```python
from build123d import *

# Parameters (mm, degrees)
REVOLVE1_ANGLE                                       = 180
BOSS_EXTRUDE1_DEPTH                                  = 10
BOSS_EXTRUDE1_DEPTH_BACK                             = 10
SKETCH2_W                                            = 5
SKETCH2_H                                            = 20
CUT_EXTRUDE1_DEPTH                                   = 10
CSK_FOR_M1_6_COUNTERSUNK_FLAT_HEAD_SCREW_D           = 1.8
CSK_FOR_M1_6_COUNTERSUNK_FLAT_HEAD_SCREW_DEPTH       = 5
CSK_FOR_M1_6_COUNTERSUNK_FLAT_HEAD_SCREW_CSINK_D     = 3.6
CSK_FOR_M1_6_COUNTERSUNK_FLAT_HEAD_SCREW_CSINK_ANGLE = 90
CSK_FOR_M1_6_COUNTERSUNK_FLAT_HEAD_SCREW_TIP         = 0.540774557
CSK_FOR_M1_6_COUNTERSUNK_FLAT_HEAD_S_2_D             = 1.8
CSK_FOR_M1_6_COUNTERSUNK_FLAT_HEAD_S_2_DEPTH         = 5
CSK_FOR_M1_6_COUNTERSUNK_FLAT_HEAD_S_2_CSINK_D       = 3.6
CSK_FOR_M1_6_COUNTERSUNK_FLAT_HEAD_S_2_CSINK_ANGLE   = 90
CSK_FOR_M1_6_COUNTERSUNK_FLAT_HEAD_S_2_TIP           = 0.540774557
CSK_FOR_M1_6_COUNTERSUNK_FLAT_HEAD_S_3_D             = 1.8
CSK_FOR_M1_6_COUNTERSUNK_FLAT_HEAD_S_3_DEPTH         = 5
CSK_FOR_M1_6_COUNTERSUNK_FLAT_HEAD_S_3_CSINK_D       = 3.6
CSK_FOR_M1_6_COUNTERSUNK_FLAT_HEAD_S_3_CSINK_ANGLE   = 90
CSK_FOR_M1_6_COUNTERSUNK_FLAT_HEAD_S_3_TIP           = 0.540774557
SKETCH9_R                                            = 3
CUT_EXTRUDE2_DEPTH                                   = 3
CUT_EXTRUDE3_START                                   = -3
SKETCH10_R                                           = 3
CUT_EXTRUDE3_DEPTH                                   = 3


with BuildPart() as part:
    # Sketch1 → Revolve1 (revolve)
    with BuildSketch(Plane.XY):
        with BuildLine():
            Line((61, 170), (61, 0))
            Line((61, 0), (58, 0))
            Line((58, 0), (58, 170))
            ThreePointArc((58, 170), (41.873834296, 218.154039035), (0, 246.884627213))
            Line((0, 246.884627213), (0, 250))
            ThreePointArc((0, 250), (44.010282534, 220.301590432), (61, 170))
        make_face()
    revolve(axis=Axis((0, 0, 0), (0, 1, 0)), revolution_arc=REVOLVE1_ANGLE)

    # Sketch2 → Boss-Extrude1 (add, two sides: drawn at the far end of the back side and taken through both)
    with BuildSketch(Plane.XY.offset(-BOSS_EXTRUDE1_DEPTH_BACK)):
        with Locations((55.5, 152)):
            Rectangle(SKETCH2_W, SKETCH2_H)
        with Locations((-55.5, 152)):
            Rectangle(SKETCH2_W, SKETCH2_H)
    extrude(amount=BOSS_EXTRUDE1_DEPTH + BOSS_EXTRUDE1_DEPTH_BACK)

    # Sketch4 → Cut-Extrude1 (cut)
    with BuildSketch(Plane.XY.offset(10)):
        Polygon((-55, 162), (-56, 162), (-58, 162), (-58, 142), (-56, 142), (-55, 142), align=None)
        Polygon((55, 142), (56, 142), (58, 142), (58, 162), (56, 162), (55, 162), align=None)
    extrude(amount=-CUT_EXTRUDE1_DEPTH, mode=Mode.SUBTRACT)

    # CSK for M1.6 Countersunk Flat Head Screw
    with Locations(Plane(origin=(60.795081967, 157.001615154, -4.995799095), x_dir=(0.081898345823, 0, 0.996640687987), z_dir=(0.996640687987, 0, -0.081898345823))):
        with Locations((0, 0)):
            CounterSinkHole(CSK_FOR_M1_6_COUNTERSUNK_FLAT_HEAD_SCREW_D / 2, CSK_FOR_M1_6_COUNTERSUNK_FLAT_HEAD_SCREW_CSINK_D / 2, depth=CSK_FOR_M1_6_COUNTERSUNK_FLAT_HEAD_SCREW_DEPTH, counter_sink_angle=CSK_FOR_M1_6_COUNTERSUNK_FLAT_HEAD_SCREW_CSINK_ANGLE)
            with Locations((0, 0, -(CSK_FOR_M1_6_COUNTERSUNK_FLAT_HEAD_SCREW_DEPTH + CSK_FOR_M1_6_COUNTERSUNK_FLAT_HEAD_SCREW_TIP / 2))):  # 118° drill point
                Cone(0, CSK_FOR_M1_6_COUNTERSUNK_FLAT_HEAD_SCREW_D / 2, CSK_FOR_M1_6_COUNTERSUNK_FLAT_HEAD_SCREW_TIP, mode=Mode.SUBTRACT)

    # CSK for M1.6 Countersunk Flat Head S 2
    with Locations(Plane(origin=(60.795081967, 147.001615154, -4.995799095), x_dir=(0.081897976852, 0, 0.996640718307), z_dir=(0.996640718307, 0, -0.081897976852))):
        with Locations((0, 0)):
            CounterSinkHole(CSK_FOR_M1_6_COUNTERSUNK_FLAT_HEAD_S_2_D / 2, CSK_FOR_M1_6_COUNTERSUNK_FLAT_HEAD_S_2_CSINK_D / 2, depth=CSK_FOR_M1_6_COUNTERSUNK_FLAT_HEAD_S_2_DEPTH, counter_sink_angle=CSK_FOR_M1_6_COUNTERSUNK_FLAT_HEAD_S_2_CSINK_ANGLE)
            with Locations((0, 0, -(CSK_FOR_M1_6_COUNTERSUNK_FLAT_HEAD_S_2_DEPTH + CSK_FOR_M1_6_COUNTERSUNK_FLAT_HEAD_S_2_TIP / 2))):  # 118° drill point
                Cone(0, CSK_FOR_M1_6_COUNTERSUNK_FLAT_HEAD_S_2_D / 2, CSK_FOR_M1_6_COUNTERSUNK_FLAT_HEAD_S_2_TIP, mode=Mode.SUBTRACT)

    # CSK for M1.6 Countersunk Flat Head S 3
    with Locations(Plane(origin=(-60.795081967, 147.001615154, -4.995799095), x_dir=(0.081897976852, 0, -0.996640718307), z_dir=(-0.996640718307, 0, -0.081897976852))):
        with Locations((0, 0), (0, -10)):
            CounterSinkHole(CSK_FOR_M1_6_COUNTERSUNK_FLAT_HEAD_S_3_D / 2, CSK_FOR_M1_6_COUNTERSUNK_FLAT_HEAD_S_3_CSINK_D / 2, depth=CSK_FOR_M1_6_COUNTERSUNK_FLAT_HEAD_S_3_DEPTH, counter_sink_angle=CSK_FOR_M1_6_COUNTERSUNK_FLAT_HEAD_S_3_CSINK_ANGLE)
            with Locations((0, 0, -(CSK_FOR_M1_6_COUNTERSUNK_FLAT_HEAD_S_3_DEPTH + CSK_FOR_M1_6_COUNTERSUNK_FLAT_HEAD_S_3_TIP / 2))):  # 118° drill point
                Cone(0, CSK_FOR_M1_6_COUNTERSUNK_FLAT_HEAD_S_3_D / 2, CSK_FOR_M1_6_COUNTERSUNK_FLAT_HEAD_S_3_TIP, mode=Mode.SUBTRACT)

    # Sketch9 → Cut-Extrude2 (cut)
    with BuildSketch(Plane(origin=(-53, 0, 0), x_dir=(0, 0, -1), z_dir=(1, 0, 0))):
        with Locations((0, 152)):
            Circle(SKETCH9_R)
    extrude(amount=-CUT_EXTRUDE2_DEPTH, mode=Mode.SUBTRACT)

    # Sketch10 → Cut-Extrude3 (cut)
    with BuildSketch(Plane.ZY.offset(-53).offset(CUT_EXTRUDE3_START)):
        with Locations(Location((0, 152, 0), (0, 0, 180))):
            Circle(SKETCH10_R)
    extrude(amount=CUT_EXTRUDE3_DEPTH, mode=Mode.SUBTRACT)


solid = part.part
```
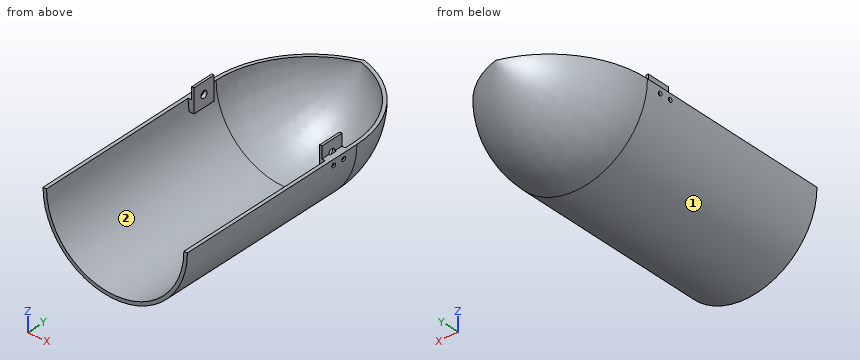
Can you work these out from the model? Positions are in its coordinate system, mm. Face numbers are marked on the shaded views. Coordinates: 2 decimals unless noted, no trailing zeros. Write each loop counter-clockwise with the first axis right and the second up, starting at its lowest first coordinate (ties: lowest second). Pieces come first, ordered by that corner, then holes. Notation, with made-up numbers: (62, 28) - (119, 28) arc R30 cw to (119, 65) - close; hole circle Ø11 at (7.25, -6). An arc over 180 degrees is marked (long way). Return JSON: item names as keys, results as strings.
Q1. If we section it at B-B (y = 41): Please give me the cut outline in (x, z), then the cut area to 3 significant figures.
Computed values:
{"outline": "(-61, 0) arc R61 ccw to (61, 0) - (58, 0) arc R58 cw to (-58, 0) - close", "area": "561 mm2"}
Q2. If we section it at A-A (y = 152): Please give me the cut outline in (x, z).
Computed values:
{"outline": "(-61, 0) arc R61 ccw to (61, 0) - (56, 0) - (56, -3) - (53, -3) - (53, -10) - (57.13, -10) arc R58 cw to (-57.13, -10) - (-53, -10) - (-53, -3) - (-56, -3) - (-56, 0) - close; (-55, 3) - (-53, 3) - (-53, 10) - (-55, 10) - close; (53, 3) - (55, 3) - (55, 10) - (53, 10) - close"}
Q3. I'm going to push flat-ended pins straight in: pin 1 Ø1 at (x, y) = (2.5, 36.5) entering from -Z; pin 2 Ø4 at (x, z) = (54.5, 1.5) entering from -Y; pin 3 Ø2 at (x, y) = (-38.5, 123) entering from -Z; pin 4 Ø22 at (y, z) = (148, -4) entering from +X. Where does each tip first touch, or does it pass through?
Computed values:
{"pin 1": "stops at z = -60.97", "pin 2": "stops at y = 142", "pin 3": "stops at z = -48.11", "pin 4": "stops at x = 61"}
Q4. Thinking about a two-plate mould opening in X: for the marked faces 1 and 2, which applies, +X half, -X half, draft (parallel to the pull), parting line (faces both ways), or undercut?
Computed values:
{"face 1": "parting line", "face 2": "undercut"}
Q5. Please list where these lines run through material, in increasing order: L1, parallel to X at y = 93.5, z = -47; L2, parallel to X at y = 196, z = -17; L3, parallel to Y at x = -8.5, z = -28. Write a range as from..to.
Computed values:
{"L1": "x = -38.88..-33.99, 33.99..38.88", "L2": "x = -54.22..-50.89, 50.89..54.22", "L3": "y = 231.4..235.26"}
